Could you check a few things on this model? Use its own coordinates, in mm. Face numbers are marked on the shaded views. Round coordinates to 2 decimals unless told otherwise and drop trailing zeros. Loops run counter-clockwise (first coordinate to the right, second up) from the corner with the lowest first, then second, coordinate; pieces in that order, holes last. Notation, with made-up numbers: (-34, 69) -> (-9, 69) arc R18 ccw to (-9, 93) -> close; hole circle Ø6 at (42, 77.25). An arc over 180 degrees is marked (long way). Put each result on its own line as item: value. Start each with the question number.
1. I'm going to push flat-ended pins straight in: P1, Ø6, axis at y = 5.5, z = 21.5, coming from the -X side; P2, Ø1, axis at x = 14, z = 11.5, coming from the +Y side; P3, Ø10, axis at x = -2, z = 12, coming from the -Y side; P4, Ø16, axis at x = 0, y = 0, coming from the -Z side. Where does each tip first touch, or does it pass through?
2. Imagine slicing it at C-C, the plane z = 5.75. Please give me the cut outline in (x, y).
3. I need wall thicknesses on line 1 (Y direction, x = 0, z = 18.75); line 2 (Y direction, x = -1, z = 11.5); line 3 (Y direction, x = -15, z = 21.5). Which ranges of each line are inside material? Lowest first, please. Write a range as [from, to].
4. Imagine slicing it at A-A, the plane y = 0. Please give me the cut outline in (x, z).
5. If we mould it in two halves opening along X, with no side actions, what happens to the marked faces 1, 2 and 3? For each: pulls with the +X half, pulls with the -X half, needs draft (parallel to the pull), parting line crosses it, or undercut.
```python
from build123d import *

# Parameters (mm, degrees)
SKIZZE1_R                       = 24
AUFSATZ_LINEAR_AUSTRAGEN1_DEPTH = 24
VERRUNDUNG1_R                   = 5
SKIZZE2_R                       = 5
SCHNITT_LINEAR_AUSTRAGEN1_DEPTH = 25


with BuildPart() as part:
    # Skizze1 → Aufsatz-Linear austragen1 (new body)
    with BuildSketch(Plane.XY):
        Circle(SKIZZE1_R)
    extrude(amount=AUFSATZ_LINEAR_AUSTRAGEN1_DEPTH)

    # Verrundung1
    verrundung1_edges = [part.edges().sort_by_distance(p)[0] for p in [
        (-24, 0, 0),
        (-24, 0, 24),
    ]]
    fillet(verrundung1_edges, radius=VERRUNDUNG1_R)

    # Skizze2 → Schnitt-Linear austragen1 (cut, through all)
    with BuildSketch(Plane(origin=(0, 0, 0), x_dir=(-1, 0, 0), z_dir=(0, 0, -1))):
        Circle(SKIZZE2_R)
    extrude(amount=-SCHNITT_LINEAR_AUSTRAGEN1_DEPTH, mode=Mode.SUBTRACT)


solid = part.part
```
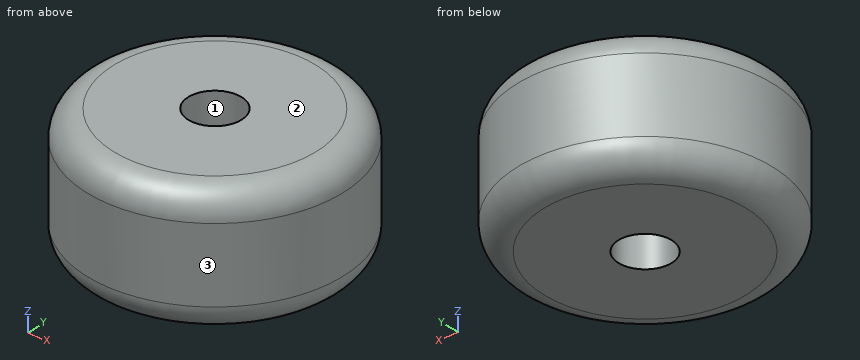
Entries:
1. P1: x = -23.75
1. P2: y = 19.84
1. P3: y = -24
1. P4: z = 0
2. outline: circle Ø48 at (0, 0); hole circle Ø10 at (0, 0)
3. line 1: [-24, -5], [5, 24]
3. line 2: [-23.98, -4.9], [4.9, 23.98]
3. line 3: [-17.87, 17.87]
4. outline: (-24, 5) arc R5 ccw to (-19, 0) -> (-5, 0) -> (-5, 24) -> (-19, 24) arc R5 ccw to (-24, 19) -> close; (5, 0) -> (19, 0) arc R5 ccw to (24, 5) -> (24, 19) arc R5 ccw to (19, 24) -> (5, 24) -> close
5. face 1: undercut
5. face 2: needs draft
5. face 3: parting line crosses it
